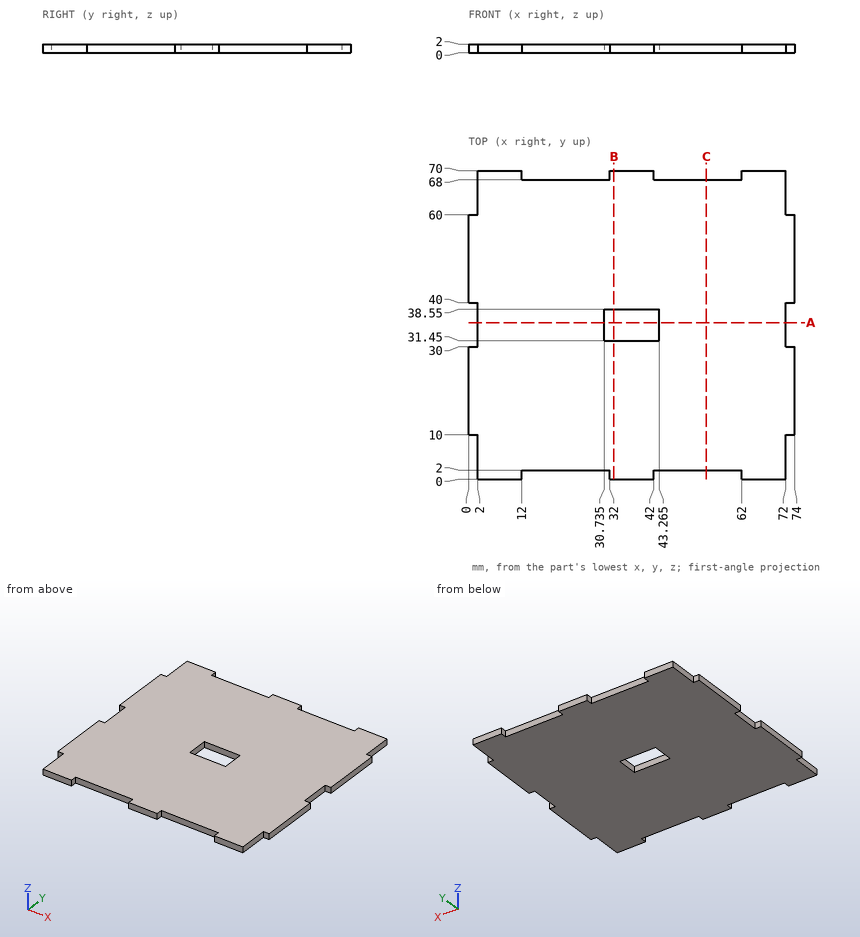
Study the drawing (mm; zero at the part's minimum x, y, z) and answer. Round coordinates to 2 decimals unless told otherwise and drop trailing zeros. Loops run counter-clockwise (first coordinate to the right, second up) from the corner with the lowest first, then second, coordinate; pieces in that order, holes last.
Q1. Section A-A, the plane y = 35.5 is taken. Determine the outline of the cut face in (x, z) (3 decimals).
Q2. Given pin 1 Ø1 at (y, z) = (4.5, 1) entering from +X; pin 2 Ø0.6 at (x, z) = (1.5, 1) entering from -Y; pin 3 Ø0.6 at (x, z) = (72.5, 1) entering from +Y, each flat-ended and moving along its own axis, determine where each tip first touches the part or whether it passes through.
Q3. Section B-B, the plane x = 33 is taken. Determine the outline of the cut face in (y, z).
Q4. Section C-C, the plane x = 54 is taken. Determine the outline of the cut face in (y, z).
Q5. Find the intervals of material crossed by line 1 (Y direction, x = 39.5, z = 0.1); line 2 (Y direction, x = 43, z = 0.1); line 3 (X direction, y = 33.5, z = 0.25) (3 decimals), in increasing order.
Completed:
1. outline: (2, 0) - (30.735, 0) - (30.735, 2) - (2, 2) - close; (43.265, 0) - (72, 0) - (72, 2) - (43.265, 2) - close
2. pin 1: stops at x = 72
2. pin 2: stops at y = 10
2. pin 3: stops at y = 60
3. outline: (0, 0) - (31.45, 0) - (31.45, 2) - (0, 2) - close; (38.55, 0) - (70, 0) - (70, 2) - (38.55, 2) - close
4. outline: (2, 0) - (68, 0) - (68, 2) - (2, 2) - close
5. line 1: y = 0 to 31.45, 38.55 to 70
5. line 2: y = 2 to 31.45, 38.55 to 68
5. line 3: x = 2 to 30.735, 43.265 to 72
